Verification items for this drawing (mm, ordinates from the low corner). A direction names the side the tool comes from. Round coordinates to 2 decimals unless told otherwise and drop trailing zeros. Write each loop counter-clockwise with the first axis right and the second up, starting at its lowest first coordinate (ties: lowest second). Pieces come first, ordered by that corner, then holes. Notation, with made-up numbers: (47, 45.25) -> (71, 45.25) arc R23 cw to (71, 69.25) -> close; hole circle Ø5 at (78.5, 58). An arc over 180 degrees is marked (long way). Put each result on its own line as item: value. Start each with the question number.
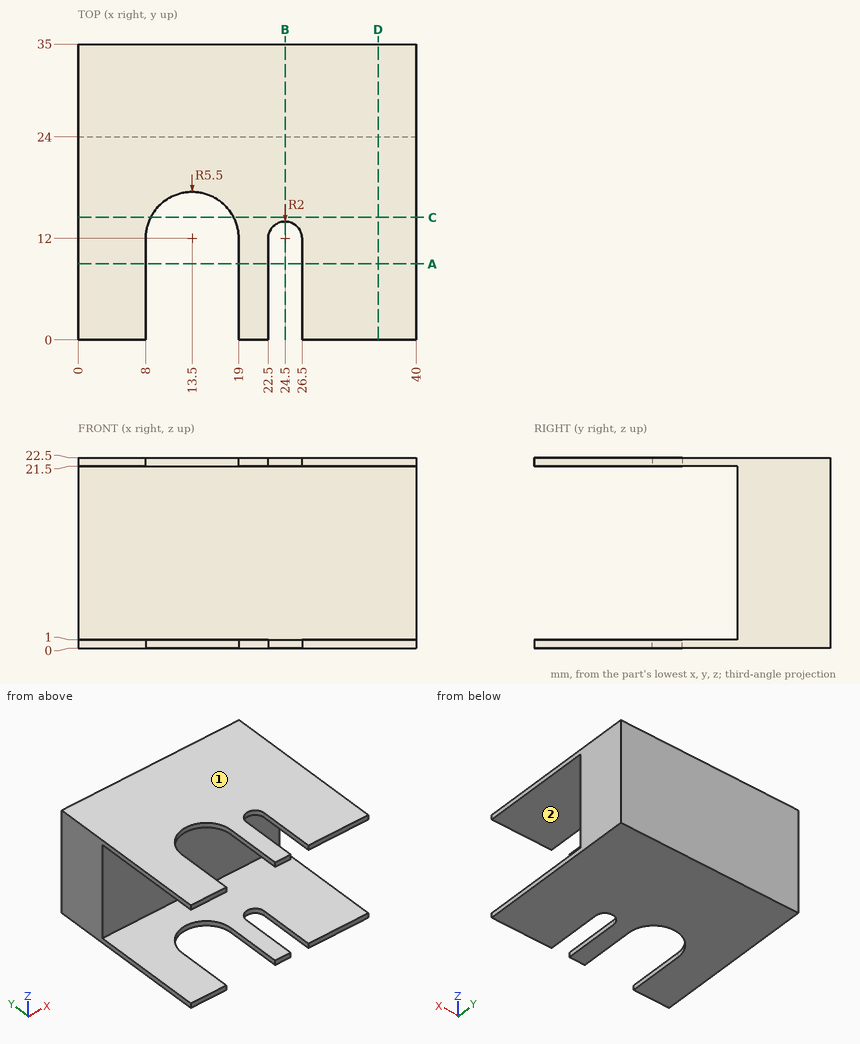
1. Section check C-C, the plane y = 14.5. Enter the section's corners in (x, z), then the cut area to 3 significant figures.
2. Section check A-A, the plane y = 9. Enter the section's corners in (x, z), then the cut area to 3 significant figures.
3. Section check D-D, the plane x = 35.5. Enter the section's corners in (y, z), then the cut area to 4 significant figures.
4. Section check B-B, the plane x = 24.5. Enter the section's corners in (y, z).
5. Access from +Z, -Z, +X, -X, +Y, -Y to the whole of each face (thin tool, end or side, straight path). Record for the marked faces 1 and 2.
6. Material ranges on L1, parallel to Z at x = 2.5, y = 14.5; L2, parallel to Y at x = 17.5, z = 4.5, recorded low to high. Write a range as [from, to].
7. Gauge pin test, flat ends, axial feed: P1, Ø12, axis at x = 18, y = 16.5, coming from the -Z side; P2, Ø6, axis at x = 19, z = 16, coming from the -Y side. Record the tip position at first contact, or that the pin passes through.
Reply:
1. outline: (0, 0) -> (8.6, 0) -> (8.6, 1) -> (0, 1) -> close; (0, 21.5) -> (8.6, 21.5) -> (8.6, 22.5) -> (0, 22.5) -> close; (18.4, 0) -> (40, 0) -> (40, 1) -> (18.4, 1) -> close; (18.4, 21.5) -> (40, 21.5) -> (40, 22.5) -> (18.4, 22.5) -> close
1. area: 60.4 mm2
2. outline: (0, 0) -> (8, 0) -> (8, 1) -> (0, 1) -> close; (0, 21.5) -> (8, 21.5) -> (8, 22.5) -> (0, 22.5) -> close; (19, 0) -> (22.5, 0) -> (22.5, 1) -> (19, 1) -> close; (19, 21.5) -> (22.5, 21.5) -> (22.5, 22.5) -> (19, 22.5) -> close; (26.5, 0) -> (40, 0) -> (40, 1) -> (26.5, 1) -> close; (26.5, 21.5) -> (40, 21.5) -> (40, 22.5) -> (26.5, 22.5) -> close
2. area: 50.0 mm2
3. outline: (0, 0) -> (35, 0) -> (35, 22.5) -> (0, 22.5) -> (0, 21.5) -> (24, 21.5) -> (24, 1) -> (0, 1) -> close
3. area: 295.5 mm2
4. outline: (14, 0) -> (35, 0) -> (35, 22.5) -> (14, 22.5) -> (14, 21.5) -> (24, 21.5) -> (24, 1) -> (14, 1) -> close
5. face 1: +Z, +X, -X, +Y, -Y
5. face 2: +X, -X, -Y
6. L1: z = [0, 1], [21.5, 22.5]
6. L2: y = [24, 35]
7. P1: stops at z = 0
7. P2: stops at y = 24
